```python
from build123d import *

# Parameters (mm, degrees)
F1_DEPTH = 10.16
F2_R     = 3.175
F3_DEPTH = 25.4
F4_W     = 12.7
F4_H     = 12.7
F5_DEPTH = 25.4


with BuildPart() as f1:
    # F0 (on Top) → F1 (new body)
    with BuildSketch(Plane.XY):
        Polygon((-38.1, 152.4), (-38.1, -76.2), (-38.1, -152.4), (38.1, -152.4), (38.1, -76.2), (38.1, 152.4), align=None)
    extrude(amount=F1_DEPTH)

    # F2 (on face) → F3 (cut)
    with BuildSketch(Plane.XY.offset(10.16)):
        with Locations((25.4, 139.7)):
            Circle(F2_R)
        with Locations((-25.4, 139.7)):
            Circle(F2_R)
    extrude(amount=-F3_DEPTH, mode=Mode.SUBTRACT)

    # F4 (on face) → F5 (join)
    with BuildSketch(Plane(origin=(0, 0, 0), x_dir=(1, 0, 0), z_dir=(0, 0, -1))):
        with Locations((0, -127)):
            Rectangle(F4_W, F4_H)
    extrude(amount=F5_DEPTH)


solid = f1.part
```
Geometry: final body of the model. Coordinates: model frame, mm. A direction names the side the tool comes from. Coordinates: 2 decimals unless noted, no trailing zeros. Order: outer loops, then holes, each group sorted by start corner. A loop starts at its lowest first (then second) coordinate and runs counter-clockwise, first axis right, second up. Notation, with made-up numbers: M 66,53.25 L 94,53.25 A27 ccw 94,90.25 Z; hole C -17,63.25 d11. An arc over 180 degrees is marked long. Answer in a Markdown table with one row per item. Add a question column.
Q1. Contact query for flat-ended pins moving along their axis: P1, Ø6, axis at x = -8, z = -14.5, coming from the -Y side; P2, Ø12, axis at x = 18, z = -16.5, coming from the -Y side; P3, Ø12, axis at x = 27, y = -102, coming from the -Z side; P4, Ø4, axis at x = -1.5, z = -9, coming from the +Y side. Output: stop coordinate, or through.
Q2. Mould query, pull axis X, two halves, no side actions, for faces 3 (the flat face through (-6.35, 127, -13)), 4 (the flat face through (0, 133.35, -13)), 5 (the flat face through (6.35, 127, -13)), 6 (the cylindrical face through (-22.37, 140.65, 5.15)). Classes: released by +X, released by -X, zero draft, split by the parting line, or undercut.
Q3. Line query: L1, parallel to Y at x = -25.4, z = 5.25 (3 decimals); L2, parallel to X at y = 139.7, z = 3 (3 decimals); L3, parallel to Y at x = 25, z = 4. Output: solid intervals per line, ascending.
Q4. Section query D-D on z = -21. Return the cut outline in (x, y).
Q5. Section query B-B on x = 25.4. Return the cut outline in (y, z) (3 decimals), and give its area (3 significant figures).
Q6. Section query C-C on x = -1.5. Return the cut outline in (y, z).
Q7. Section query A-A on y = 139.7. Return the cut outline in (x, z) (3 decimals), and give its area (3 significant figures).
Q8. Reachability of faces 1 (the flat face through (38.1, -2, 5)), 2 (the flat face through (0, 120.65, -13)) from +Z, -Z, +X, -X, +Y, -Y: full face, straight path, thin tool, end or side. Return the list, or none.
Completed:
| question | item | result |
|---|---|---|
| 1 | P1 | stops at y = 120.65 |
| 1 | P2 | passes through |
| 1 | P3 | stops at z = 0 |
| 1 | P4 | stops at y = 133.35 |
| 2 | face 3 | released by -X |
| 2 | face 4 | zero draft |
| 2 | face 5 | released by +X |
| 2 | face 6 | undercut |
| 3 | L1 | y = -152.4 to 136.525, 142.875 to 152.4 |
| 3 | L2 | x = -38.1 to -28.575, -22.225 to 22.225, 28.575 to 38.1 |
| 3 | L3 | y = -152.4 to 136.55, 142.85 to 152.4 |
| 4 | outline | M -6.35,120.65 L 6.35,120.65 L 6.35,133.35 L -6.35,133.35 Z |
| 5 | outline | M -152.4,0 L 136.525,0 L 136.525,10.16 L -152.4,10.16 Z; M 142.875,0 L 152.4,0 L 152.4,10.16 L 142.875,10.16 Z |
| 5 | area | 3,030 mm2 |
| 6 | outline | M -152.4,0 L 120.65,0 L 120.65,-25.4 L 133.35,-25.4 L 133.35,0 L 152.4,0 L 152.4,10.16 L -152.4,10.16 Z |
| 7 | outline | M -38.1,0 L -28.575,0 L -28.575,10.16 L -38.1,10.16 Z; M -22.225,0 L 22.225,0 L 22.225,10.16 L -22.225,10.16 Z; M 28.575,0 L 38.1,0 L 38.1,10.16 L 28.575,10.16 Z |
| 7 | area | 645 mm2 |
| 8 | face 1 | +Z, -Z, +X, +Y, -Y |
| 8 | face 2 | -Z, +X, -X, -Y |
